Here's the drawing with two shaded views (mm, measured from the low corner). I have some questions. A direction names the side the tool comes from. Coordinates: 2 decimals unless noted, no trailing zeros. Write each loop counter-clockwise with the first axis right and the second up, starting at its lowest first coordinate (ties: lowest second). Pieces come first, ordered by that corner, then holes. Notation, with made-up numbers: (28, 14.25) -> (85, 14.25) arc R27 cw to (85, 31.25) -> close; hole circle Ø5 at (61.25, 77.5). An arc over 180 degrees is marked (long way). Answer in a Markdown table with one row per item. Add a question column.
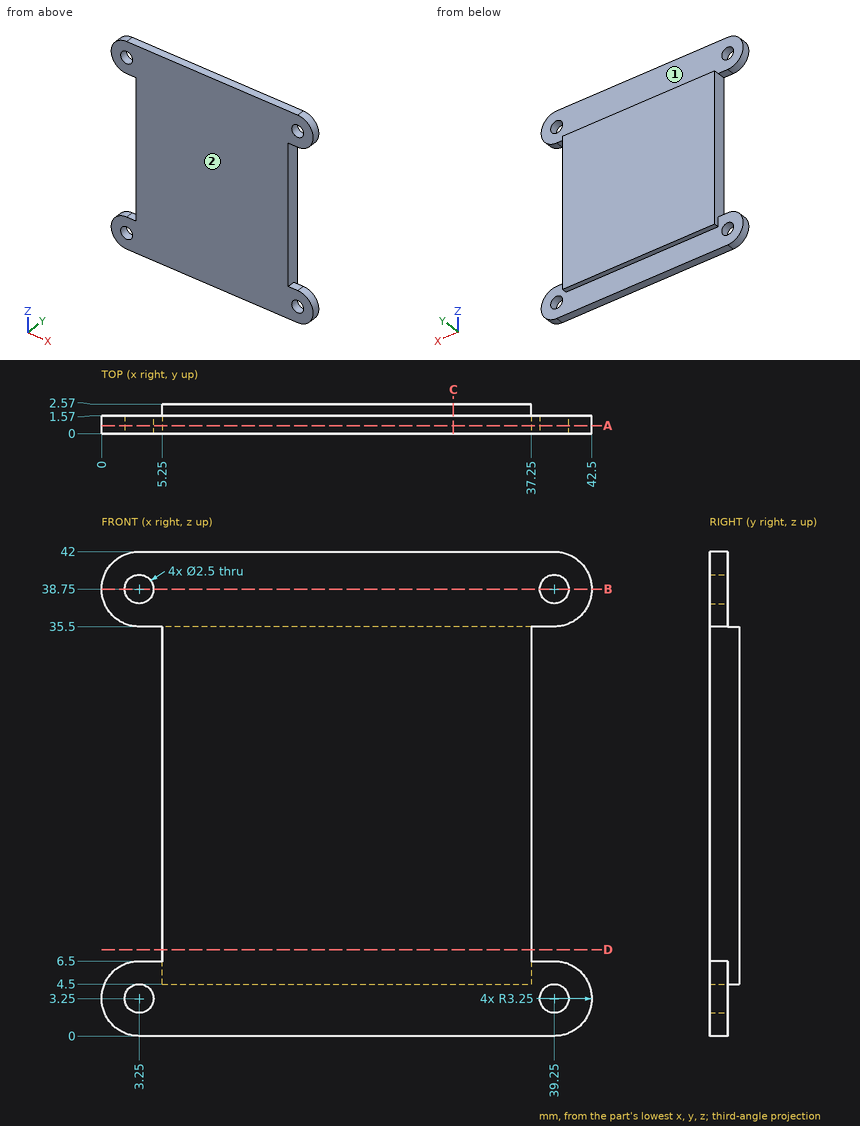
Q1. Imagine slicing it at D-D on z = 7.5. Please give me the cut outline in (x, y).
Q2. Imagine slicing it at B-B on z = 38.75. Please give me the cut outline in (x, y), plus the area to 3 significant figures.
Q3. For the marked faces 1 and 2, which set-ups out of +Z, -Z, +X, -X, +Y, -Y let a thin tool reach every point of the face, with its end or its side?
Q4. Imagine slicing it at C-C on x = 30.5. Please give me the cut outline in (y, z).
Q5. I need wall thicknesses on line 1 (Z direction, x = 39.25, y = 0.8); line 2 (X direction, y = 0.95, z = 15); line 3 (Z direction, x = 20.5, y = 2.3). Which ranges of each line are inside material? Lowest first, please. Write a range as [from, to].
Q6. I'm going to push flat-ended pins straight in: P1, Ø0.8, axis at x = 4, y = 0.5, coming from the -Z side; P2, Ø5, axis at x = 27.5, z = 40, coming from the +Y side; P3, Ø1, axis at y = 1, z = 37.5, coming from the +X side; P4, Ø1.1, axis at x = 28, y = 2.5, coming from the -Z side. Where does each tip first touch, or does it pass through?
Q7. Imagine slicing it at A-A on y = 0.7. Please give me the cut outline in (x, z), plus the area to 3 significant figures.
Result sheet:
| question | item | result |
|---|---|---|
| 1 | outline | (5.25, 0) -> (37.25, 0) -> (37.25, 2.57) -> (5.25, 2.57) -> close |
| 2 | outline | (0, 0) -> (2, 0) -> (2, 1.57) -> (0, 1.57) -> close; (4.5, 0) -> (38, 0) -> (38, 1.57) -> (4.5, 1.57) -> close; (40.5, 0) -> (42.5, 0) -> (42.5, 1.57) -> (40.5, 1.57) -> close |
| 2 | area | 58.9 mm^2 |
| 3 | face 1 | +Z, +X, -X, +Y |
| 3 | face 2 | +Z, -Z, +X, -X, -Y |
| 4 | outline | (0, 0) -> (1.57, 0) -> (1.57, 4.5) -> (2.57, 4.5) -> (2.57, 35.5) -> (1.57, 35.5) -> (1.57, 42) -> (0, 42) -> close |
| 5 | line 1 | z = [0, 2], [4.5, 6.5], [35.5, 37.5], [40, 42] |
| 5 | line 2 | x = [5.25, 37.25] |
| 5 | line 3 | z = [4.5, 35.5] |
| 6 | P1 | stops at z = 0 |
| 6 | P2 | stops at y = 1.57 |
| 6 | P3 | stops at x = 42.41 |
| 6 | P4 | stops at z = 4.5 |
| 7 | outline | (3.25, 0) -> (39.25, 0) arc R3.25 ccw to (39.25, 6.5) -> (37.25, 6.5) -> (37.25, 35.5) -> (39.25, 35.5) arc R3.25 ccw to (39.25, 42) -> (3.25, 42) arc R3.25 ccw to (3.25, 35.5) -> (5.25, 35.5) -> (5.25, 6.5) -> (3.25, 6.5) arc R3.25 ccw to start; hole circle Ø2.5 at (3.25, 3.25); hole circle Ø2.5 at (3.25, 38.75); hole circle Ø2.5 at (39.25, 3.25); hole circle Ø2.5 at (39.25, 38.75) |
| 7 | area | 1,440 mm^2 |
